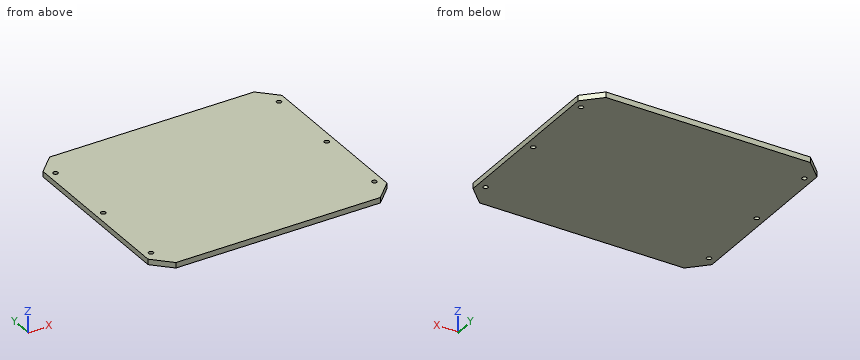
from build123d import *

# Parameters (mm, degrees)
SKETCH1_W           = 278
SKETCH1_H           = 238
BOSS_EXTRUDE1_DEPTH = 6.35
CHAMFER1_SIZE       = 20
SKETCH4_R           = 2.75
CUT_EXTRUDE2_DEPTH  = 76.2


with BuildPart() as part:
    # Sketch1 → Boss-Extrude1 (new body)
    with BuildSketch(Plane.XY):
        Rectangle(SKETCH1_W, SKETCH1_H)
    extrude(amount=BOSS_EXTRUDE1_DEPTH)

    # Chamfer1
    chamfer1_edges = [part.edges().sort_by_distance(p)[0] for p in [
        (-139, 119, 3.175),
        (139, 119, 3.175),
        (139, -119, 3.175),
        (-139, -119, 3.175),
    ]]
    chamfer(chamfer1_edges, length=CHAMFER1_SIZE)

    # Sketch4 → Cut-Extrude2 (cut)
    with BuildSketch(Plane.XY.offset(6.35)):
        with Locations((-130, 90)):
            Circle(SKETCH4_R)
        with Locations((-130, -90)):
            Circle(SKETCH4_R)
        with Locations((-130, 0)):
            Circle(SKETCH4_R)
        with Locations((130, -90)):
            Circle(SKETCH4_R)
        with Locations((130, 0)):
            Circle(SKETCH4_R)
        with Locations((130, 90)):
            Circle(SKETCH4_R)
    extrude(amount=-CUT_EXTRUDE2_DEPTH, mode=Mode.SUBTRACT)


solid = part.part
The model under review builds one solid part; all positions refer to its coordinate system, in mm. Coordinates: 2 decimals unless noted, no trailing zeros. Loops run counter-clockwise (first coordinate to the right, second up) from the corner with the lowest first, then second, coordinate; pieces in that order, holes last. Notation, with made-up numbers: (29.25, 74) -> (54.25, 74) arc R16 ccw to (54.25, 88) -> close; hole circle Ø3 at (38.5, 65). An arc over 180 degrees is marked (long way). Use a Markdown table: item, result. Add a question column.
1. To check wall thickness, follow line 1 (Y direction, x = -130, z = 2.5); line 2 (X direction, y = -0.5, z = 5.75); line 3 (X direction, y = -102.5, z = 0.75). State the ranges of each line that lie inside material, in increasing order.
2. Clearance check with a flat-ended pin moving along its axis: pin 1 Ø3 at (x, y) = (85.5, 86.5) entering from -Z. State where the tip first meets the part, or that it passes through.
3. Add section A-A on y = 104. Write out the cut boundary in (x, z), plus the area to 3 significant figures.
Returned:
| question | item | result |
|---|---|---|
| 1 | line 1 | y = -108 to -92.75, -87.25 to -2.75, 2.75 to 87.25, 92.75 to 108 |
| 1 | line 2 | x = -139 to -132.7, -127.3 to 127.3, 132.7 to 139 |
| 1 | line 3 | x = -135.5 to 135.5 |
| 2 | pin 1 | stops at z = 0 |
| 3 | outline | (-134, 0) -> (134, 0) -> (134, 6.35) -> (-134, 6.35) -> close |
| 3 | area | 1,700 mm² |
